Model file for the job. Use its own axes, mm. Face numbers are marked on the shaded views. A direction names the side the tool comes from. Round coordinates to 2 decimals unless told otherwise and drop trailing zeros. Order: outer loops, then holes, each group sorted by start corner. A loop starts at its lowest first (then second) coordinate and runs counter-clockwise, first axis right, second up. Notation, with made-up numbers: M 30,-35.75 L 67,-35.75 A27 ccw 67,-15.75 Z; hole C 55,30.25 d5. An arc over 180 degrees is marked long. Return JSON: item names as keys, results as strings. Group by question number.
Item 1: Pin check, flat tips, straight feed: pin 1 Ø4 at (y, z) = (19, 23.5) entering from +X; pin 2 Ø6 at (x, z) = (27, 13) entering from +Y; pin 3 Ø1.5 at (y, z) = (43.5, 8) entering from +X. Stop position of each tip, or through.
Item 2: Slice it at D-D on y = 35.5. Write the cut outline in (x, z), then the cut area to 4 significant figures.
Item 3: Slice it at A-A on z = 14. Write the cut outline in (x, y), then the cut area to 3 significant figures.
Item 4: Pull direction Z, two halves, no side cores. Call the marked faces 4, 5 and 6: pulls with the +Z half, pulls with the -Z half, needs draft (parallel to the pull), parting line crosses it, or undercut.
Item 5: Slice it at C-C on x = 12.5. Write the cut outline in (y, z), then the cut area to 4 significant figures.
Item 6: Probe line 1 along Y through (x, z) = (33.5, 10.75); line 2 along Z through (x, y) = (3, 15.5). List the from-to ranges inside material, lowest first.
Item 7: Slice it at B-B on y = 11. Write the cut outline in (x, z).
Item 8: Which spindle directions (+Z, -Z, +X, -X, +Y, -Y) get a long thin tool onto all of the face, cutting with end or side? Do the marked faces 1, 2 and 3. Say none if no direction does.
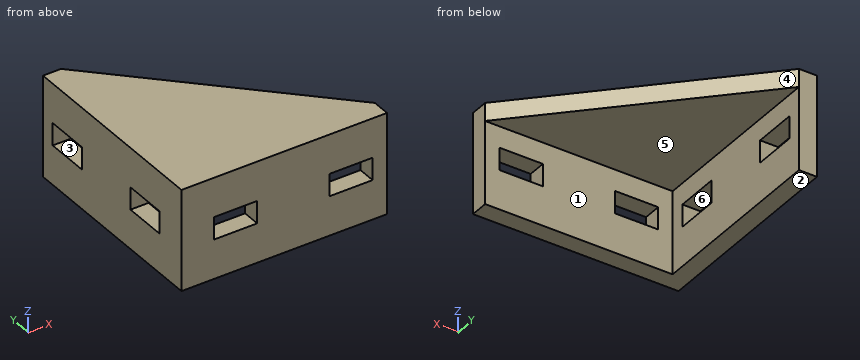
from build123d import *

# Parameters (mm, degrees)
BOSS_EXTRUDE1_DEPTH = 28
BOSS_EXTRUDE2_DEPTH = 5
SKETCH3_W           = 6.2
SKETCH3_H           = 12
CUT_EXTRUDE1_DEPTH  = 5
SKETCH4_W           = 12
SKETCH4_H           = 6.2
CUT_EXTRUDE2_DEPTH  = 5


with BuildPart() as part:
    # Sketch1 → Boss-Extrude1 (new body)
    with BuildSketch(Plane.XY):
        Polygon((5, 57), (5, 5), (57, 5), (57, 0), (0, 0), (0, 57), align=None)
    extrude(amount=BOSS_EXTRUDE1_DEPTH)

    # Sketch2 → Boss-Extrude2 (add)
    with BuildSketch(Plane.XY.offset(28)):
        Polygon((5, 57), (57, 5), (5, 5), align=None)
    extrude(amount=-BOSS_EXTRUDE2_DEPTH)

    # Sketch3 → Cut-Extrude1 (cut)
    with BuildSketch(Plane(origin=(5, 0, 0), x_dir=(0, 0, -1), z_dir=(1, 0, 0))):
        with Locations((-14, 47)):
            Rectangle(SKETCH3_W, SKETCH3_H)
        with Locations((-14, 15)):
            Rectangle(SKETCH3_W, SKETCH3_H)
    extrude(amount=-CUT_EXTRUDE1_DEPTH, mode=Mode.SUBTRACT)

    # Sketch4 → Cut-Extrude2 (cut)
    with BuildSketch(Plane(origin=(0, 5, 0), x_dir=(1, 0, 0), z_dir=(0, 1, 0))):
        with Locations((47, -14)):
            Rectangle(SKETCH4_W, SKETCH4_H)
        with Locations((15, -14)):
            Rectangle(SKETCH4_W, SKETCH4_H)
    extrude(amount=-CUT_EXTRUDE2_DEPTH, mode=Mode.SUBTRACT)


solid = part.part
Output values:
{
 "1": {"pin 1": "x = 45", "pin 2": "y = 5", "pin 3": "x = 5"},
 "2": {"outline": "M 0,0 L 5,0 L 5,23 L 26.5,23 L 26.5,28 L 0,28 Z", "area": "247.5 mm²"},
 "3": {"outline": "M 0,0 L 9,0 L 9,5 L 5,5 L 5,9 L 0,9 Z; M 0,21 L 5,21 L 5,41 L 0,41 Z; M 0,53 L 5,53 L 5,57 L 0,57 Z; M 21,0 L 41,0 L 41,5 L 21,5 Z; M 53,0 L 57,0 L 57,5 L 53,5 Z", "area": "305 mm²"},
 "4": {"face 4": "needs draft", "face 5": "pulls with the -Z half", "face 6": "undercut"},
 "5": {"outline": "M 0,0 L 5,0 L 5,10.9 L 0,10.9 Z; M 0,17.1 L 5,17.1 L 5,23 L 49.5,23 L 49.5,28 L 0,28 Z", "area": "331.5 mm²"},
 "6": {"line 1": "0 to 5", "line 2": "0 to 10.9, 17.1 to 28"},
 "7": {"outline": "M 0,0 L 5,0 L 5,10.9 L 0,10.9 Z; M 0,17.1 L 5,17.1 L 5,23 L 51,23 L 51,28 L 0,28 Z"},
 "8": {"face 1": "-Z, +X, +Y", "face 2": "-Z, +X, -X, +Y, -Y", "face 3": "+X, -X"}
}
